Geometry: final body of the model. Coordinates: model frame, mm. A direction names the side the tool comes from. Give positions to 0.01 mm unless a question says otherwise; leave off trailing zeros. Order: outer loops, then holes, each group sorted by start corner. A loop starts at its lowest first (then second) coordinate and runs counter-clockwise, first axis right, second up. Notation, with made-up numbers: (25.5, -11.5) - (37.5, -11.5) arc R7 ccw to (37.5, -5.5) - close; hole circle Ø3 at (51.25, 70). An arc over 180 degrees is marked (long way). Put each result on its own line as item: value. Start each with the question number.
1. Set-up query: faces 4 (the flat face through (-2.567, -8.619, 3.274)), 5 (the flat face through (-2.28, 0.49, -0.16)), 6 (the flat face through (-3.274, -8.619, -2.567)), 7 (the flat face through (-2.547, -8.619, -3.254)). Return all of +Z, -Z, +X, -X, +Y, -Y with unobstructed straight access to the full face (end or side cutting, diameter ignored); none if empty.
2. Mould query, pull axis X, two halves, no side actions, for faces 1 (the flat face through (-3.254, -8.619, 2.547)), 2 (the flat face through (3, -17, 3)), 3 (the flat face through (-0.16, 0.49, -2.26)). Classes: pulls with the +X half, pulls with the -X half, needs draft (parallel to the pull), parting line crosses it, or undercut.
3. First-contact query: P1, Ø1, axis at x = -6, z = -9, coming from the -Y side; P2, Ø19, axis at x = -8, z = -9, coming from the -Y side; P3, Ø5, axis at y = -6, z = -7, coming from the -X side. Flat tips, straight axial feed; report the tip coordinate or a pass-through.
4. Section C-C on x = -13.5. Return the cut outline in (y, z) (3 decimals).
5. Section A-A on y = -6.25. Return the cut outline in (x, z).
6. Ray query, line 1 along Y through (x, z) = (16.5, 1); line 2 along Z through (x, y) = (-3.5, -10.25). Return the intervals inside material, ascending. Write a range as from..to.
7. Section B-B on z = 14. Return the cut outline in (x, y) (3 decimals).
from build123d import *

# Parameters (mm, degrees)
SKETCH2_W           = 38.37
SKETCH2_H           = 38.37
BOSS_EXTRUDE6_DEPTH = 1
BOSS_EXTRUDE7_START = -17
BOSS_EXTRUDE7_DEPTH = 17


with BuildPart() as part:
    # Sketch2 → Boss-Extrude6 (new body)
    # profile 1 of 5: a face of its own
    with BuildSketch(Plane(origin=(0, 0, 0), x_dir=(1, 0, 0), z_dir=(0, 1, 0))):
        Rectangle(SKETCH2_W, SKETCH2_H)
        with BuildLine():
            Line((-3.976901657, -3.269794876), (-2.550972937, -1.843866156))
            ThreePointArc((-2.550972937, -1.843866156), (-2.22568027, -2.22568027), (-1.843866156, -2.550972937))
            Line((-1.843866156, -2.550972937), (-3.269794876, -3.976901657))
            ThreePointArc((-3.269794876, -3.976901657), (-3.640556642, -3.640556642), (-3.976901657, -3.269794876))
        make_face(mode=Mode.SUBTRACT)
        with BuildLine():
            Line((3.269794876, -3.976901657), (1.843866156, -2.550972937))
            ThreePointArc((1.843866156, -2.550972937), (2.22568027, -2.22568027), (2.550972937, -1.843866156))
            Line((2.550972937, -1.843866156), (3.976901657, -3.269794876))
            ThreePointArc((3.976901657, -3.269794876), (3.640556642, -3.640556642), (3.269794876, -3.976901657))
        make_face(mode=Mode.SUBTRACT)
        with BuildLine():
            ThreePointArc((-1.39658967, 0.097659063), (-0.989949494, 0.989949494), (-0.097659063, 1.39658967))
            Line((-0.097659063, 1.39658967), (-0.219564585, 3.139919858))
            ThreePointArc((-0.219564585, 3.139919858), (0, 3.147587223), (0.219564585, 3.139919858))
            Line((0.219564585, 3.139919858), (0.097659063, 1.39658967))
            ThreePointArc((0.097659063, 1.39658967), (0.989949494, 0.989949494), (1.39658967, 0.097659063))
            Line((1.39658967, 0.097659063), (3.139919858, 0.219564585))
            ThreePointArc((3.139919858, 0.219564585), (3.147587223, 0), (3.139919858, -0.219564585))
            Line((3.139919858, -0.219564585), (1.39658967, -0.097659063))
            ThreePointArc((1.39658967, -0.097659063), (0.989949494, -0.989949494), (0.097659063, -1.39658967))
            Line((0.097659063, -1.39658967), (0.219564585, -3.139919858))
            ThreePointArc((0.219564585, -3.139919858), (0, -3.147587223), (-0.219564585, -3.139919858))
            Line((-0.219564585, -3.139919858), (-0.097659063, -1.39658967))
            ThreePointArc((-0.097659063, -1.39658967), (-0.989949494, -0.989949494), (-1.39658967, -0.097659063))
            Line((-1.39658967, -0.097659063), (-3.139919858, -0.219564585))
            ThreePointArc((-3.139919858, -0.219564585), (-3.147587223, 0), (-3.139919858, 0.219564585))
            Line((-3.139919858, 0.219564585), (-1.39658967, 0.097659063))
        make_face(mode=Mode.SUBTRACT)
        with BuildLine():
            Line((-3.269794876, 3.976901657), (-1.843866156, 2.550972937))
            ThreePointArc((-1.843866156, 2.550972937), (-2.22568027, 2.22568027), (-2.550972937, 1.843866156))
            Line((-2.550972937, 1.843866156), (-3.976901657, 3.269794876))
            ThreePointArc((-3.976901657, 3.269794876), (-3.640556642, 3.640556642), (-3.269794876, 3.976901657))
        make_face(mode=Mode.SUBTRACT)
        with BuildLine():
            Line((3.976901657, 3.269794876), (2.550972937, 1.843866156))
            ThreePointArc((2.550972937, 1.843866156), (2.22568027, 2.22568027), (1.843866156, 2.550972937))
            Line((1.843866156, 2.550972937), (3.269794876, 3.976901657))
            ThreePointArc((3.269794876, 3.976901657), (3.640556642, 3.640556642), (3.976901657, 3.269794876))
        make_face(mode=Mode.SUBTRACT)
    # profile 2 of 5: a face of its own
    with BuildSketch(Plane(origin=(0, 0, 0), x_dir=(1, 0, 0), z_dir=(0, 1, 0))):
        with BuildLine():
            ThreePointArc((-3.269794876, -3.976901657), (-3.640556642, -3.640556642), (-3.976901657, -3.269794876))
            Line((-3.976901657, -3.269794876), (-2.550972937, -1.843866156))
            ThreePointArc((-2.550972937, -1.843866156), (-2.22568027, -2.22568027), (-1.843866156, -2.550972937))
            Line((-1.843866156, -2.550972937), (-3.269794876, -3.976901657))
        make_face()
    # profile 3 of 5: a face of its own
    with BuildSketch(Plane(origin=(0, 0, 0), x_dir=(1, 0, 0), z_dir=(0, 1, 0))):
        with BuildLine():
            Line((-2.550972937, 1.843866156), (-3.976901657, 3.269794876))
            ThreePointArc((-3.976901657, 3.269794876), (-3.640556642, 3.640556642), (-3.269794876, 3.976901657))
            Line((-3.269794876, 3.976901657), (-1.843866156, 2.550972937))
            ThreePointArc((-1.843866156, 2.550972937), (-2.22568027, 2.22568027), (-2.550972937, 1.843866156))
        make_face()
    # profile 4 of 5: a face of its own
    with BuildSketch(Plane(origin=(0, 0, 0), x_dir=(1, 0, 0), z_dir=(0, 1, 0))):
        with BuildLine():
            ThreePointArc((3.269794876, 3.976901657), (3.640556642, 3.640556642), (3.976901657, 3.269794876))
            Line((3.976901657, 3.269794876), (2.550972937, 1.843866156))
            ThreePointArc((2.550972937, 1.843866156), (2.22568027, 2.22568027), (1.843866156, 2.550972937))
            Line((1.843866156, 2.550972937), (3.269794876, 3.976901657))
        make_face()
    # profile 5 of 5: a face of its own
    with BuildSketch(Plane(origin=(0, 0, 0), x_dir=(1, 0, 0), z_dir=(0, 1, 0))):
        with BuildLine():
            ThreePointArc((3.976901657, -3.269794876), (3.640556642, -3.640556642), (3.269794876, -3.976901657))
            Line((3.269794876, -3.976901657), (1.843866156, -2.550972937))
            ThreePointArc((1.843866156, -2.550972937), (2.22568027, -2.22568027), (2.550972937, -1.843866156))
            Line((2.550972937, -1.843866156), (3.976901657, -3.269794876))
        make_face()
    extrude(amount=BOSS_EXTRUDE6_DEPTH)

    # Sketch7 → Boss-Extrude7 (add)
    with BuildSketch(Plane(origin=(0, 0, 0), x_dir=(1, 0, 0), z_dir=(0, 1, 0)).offset(BOSS_EXTRUDE7_START)):
        with BuildLine():
            Line((-3.976901657, 3.269794876), (-2.550972937, 1.843866156))
            ThreePointArc((-2.550972937, 1.843866156), (-2.22568027, 2.22568027), (-1.843866156, 2.550972937))
            Line((-1.843866156, 2.550972937), (-3.269794876, 3.976901657))
            ThreePointArc((-3.269794876, 3.976901657), (-3.640556642, 3.640556642), (-3.976901657, 3.269794876))
        make_face()
        with BuildLine():
            ThreePointArc((-1.843866156, -2.550972937), (-2.22568027, -2.22568027), (-2.550972937, -1.843866156))
            Line((-2.550972937, -1.843866156), (-3.976901657, -3.269794876))
            ThreePointArc((-3.976901657, -3.269794876), (-3.640556642, -3.640556642), (-3.269794876, -3.976901657))
            Line((-3.269794876, -3.976901657), (-1.843866156, -2.550972937))
        make_face()
        with BuildLine():
            Line((3.269794876, 3.976901657), (1.843866156, 2.550972937))
            ThreePointArc((1.843866156, 2.550972937), (2.22568027, 2.22568027), (2.550972937, 1.843866156))
            Line((2.550972937, 1.843866156), (3.976901657, 3.269794876))
            ThreePointArc((3.976901657, 3.269794876), (3.640556642, 3.640556642), (3.269794876, 3.976901657))
        make_face()
        with BuildLine():
            ThreePointArc((2.550972937, -1.843866156), (2.22568027, -2.22568027), (1.843866156, -2.550972937))
            Line((1.843866156, -2.550972937), (3.269794876, -3.976901657))
            ThreePointArc((3.269794876, -3.976901657), (3.640556642, -3.640556642), (3.976901657, -3.269794876))
            Line((3.976901657, -3.269794876), (2.550972937, -1.843866156))
        make_face()
    extrude(amount=BOSS_EXTRUDE7_DEPTH)


solid = part.part
Resolved:
1. face 4: +Z, -Y
1. face 5: +Y, -Y
1. face 6: -X, -Y
1. face 7: -Z, -Y
2. face 1: pulls with the -X half
2. face 2: needs draft
2. face 3: undercut
3. P1: y = 0
3. P2: y = -17
3. P3: through
4. outline: (0, -19.185) - (1, -19.185) - (1, 19.185) - (0, 19.185) - close
5. outline: (-3.98, -3.27) arc R5.15 ccw to (-3.27, -3.98) - (-1.84, -2.55) arc R3.15 cw to (-2.55, -1.84) - close; (-3.98, 3.27) - (-2.55, 1.84) arc R3.15 cw to (-1.84, 2.55) - (-3.27, 3.98) arc R5.15 ccw to start; (1.84, -2.55) - (3.27, -3.98) arc R5.15 ccw to (3.98, -3.27) - (2.55, -1.84) arc R3.15 cw to start; (1.84, 2.55) arc R3.15 cw to (2.55, 1.84) - (3.98, 3.27) arc R5.15 ccw to (3.27, 3.98) - close
6. line 1: 0..1
6. line 2: -3.78..-2.79, 2.79..3.78
7. outline: (-19.185, 0) - (19.185, 0) - (19.185, 1) - (-19.185, 1) - close
